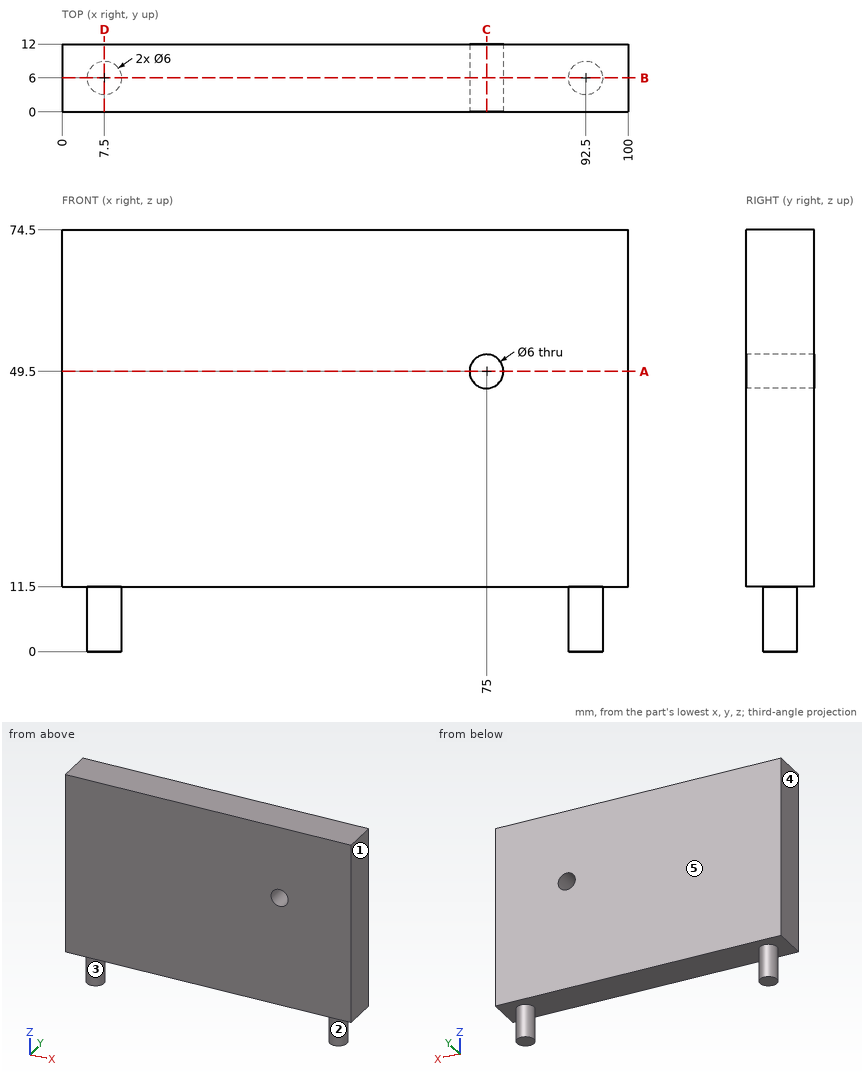
Answer from the drawing. Dimensions are ordinates in mm from the lowest x, y and z of the part. A direction names the side the tool comes from. Round coordinates to 2 decimals unless told otherwise and drop trailing zeros. Order: outer loops, then holes, each group sorted by start corner. A loop starts at its lowest first (then second) coordinate and runs counter-clockwise, first axis right, second up. Notation, with made-up numbers: (76, 31.5) -> (133, 31.5) arc R27 cw to (133, 61.5) -> close; hole circle Ø1 at (33, 72.5). An arc over 180 degrees is marked (long way). Answer as CSV lines item,"result".
Q1. A cutting plane is placed at B-B on y = 6. Determine the outline of the cut face in (x, z).
Computed values:
outline,"(0, 11.5) -> (4.5, 11.5) -> (4.5, 0) -> (10.5, 0) -> (10.5, 11.5) -> (89.5, 11.5) -> (89.5, 0) -> (95.5, 0) -> (95.5, 11.5) -> (100, 11.5) -> (100, 74.5) -> (0, 74.5) -> close; hole circle Ø6 at (75, 49.5)"
Q2. Which of the six approach directions +Z, -Z, +X, -X, +Y, -Y give full straight-line access (tool end or side, diameter ignored) to the marked faces 1 and 2?
Computed values:
face 1,"+Z, -Z, +X, +Y, -Y"
face 2,"-Z"
Q3. For a pull along X with two mould halves and no side action, classify the marked faces 3, 4 and 5 as +X half, -X half, draft (parallel to the pull), parting line (faces both ways), or undercut.
Computed values:
face 3,"undercut"
face 4,"-X half"
face 5,"draft"
Q4. A cutting plane is placed at D-D on x = 7.5. Determine the outline of the cut face in (y, z), plus the area to 3 significant figures.
Computed values:
outline,"(0, 11.5) -> (3, 11.5) -> (3, 0) -> (9, 0) -> (9, 11.5) -> (12, 11.5) -> (12, 74.5) -> (0, 74.5) -> close"
area,"825 mm^2"
Q5. Consider line 1 (Z direction, x = 75, y = 7.75); line 2 (Z direction, x = 71, y = 7.5). Determine where each line is inside the solid, lowest interval first. Write a range as from..to.
Computed values:
line 1,"z = 11.5..46.5, 52.5..74.5"
line 2,"z = 11.5..74.5"
Q6. A cutting plane is placed at C-C on x = 75. Determine the outline of the cut face in (y, z), plus the area to 3 significant figures.
Computed values:
outline,"(0, 11.5) -> (12, 11.5) -> (12, 46.5) -> (0, 46.5) -> close; (0, 52.5) -> (12, 52.5) -> (12, 74.5) -> (0, 74.5) -> close"
area,"684 mm^2"
Q7. A cutting plane is placed at A-A on z = 49.5. Determine the outline of the cut face in (x, y).
Computed values:
outline,"(0, 0) -> (72, 0) -> (72, 12) -> (0, 12) -> close; (78, 0) -> (100, 0) -> (100, 12) -> (78, 12) -> close"
Q8. Given pin 1 (3 mm diameter, centred on x = 46.5, y = 2, fed in from -Z), flat-ended and moving along its own axis, determine where the tip first touches the part or whether it passes through.
Computed values:
pin 1,"stops at z = 11.5"
